Design review of the part shown in the three views and the two pictorial views. Dimensions are in mm from the part's minimum x, y and z. A direction names the side the tool comes from. Round coordinates to 2 decimals unless told otherwise and drop trailing zeros. Loops run counter-clockwise (first coordinate to the right, second up) from the corner with the lowest first, then second, coordinate; pieces in that order, holes last.
1) Take a section at D-D (z = 26). State the section outline as (x, y) points, then the cut area to 3 significant figures.
2) Wall thickness on L1, parallel to Y at x = 13.65, z = 3.5; L2, parallel to X at y = 25.75, z = 4; L3, parallel to Z at x = 8.75, y = 11.25: over which ranges is each line inside the solid? List them lowest first.
3) Take a section at A-A (z = 30.5). State the section outline as (x, y) points.
4) Take a section at C-C (y = 9.25). State the section outline as (x, z) points.
5) Tool access review of the marked faces 1, 2 and 3: name each direction out of +Z, -Z, +X, -X, +Y, -Y from which nothing blocks a thin tool from reaching the whole face with its end or side.
6) Take a section at B-B (y = 15). State the section outline as (x, z) points.
7) Mouldability with a two-part tool opening along X and no side actions: class the marked faces 4, 5 and 6 as pulls with the +X half, pulls with the -X half, needs draft (parallel to the pull), parting line crosses it, or undercut.
8) Insertion check: pin 1 (3.5 mm diameter, centred on x = 8, y = 17, fed in from +Z); pin 2 (6 mm diameter, centred on x = 5, z = 16, fed in from +Y); pin 3 (6 mm diameter, centred on x = 4.5, z = 16.5, fed in from -Y). Each pin has a flat end and moves straight along its axis. Give the tip position at first contact, or say it passes through.
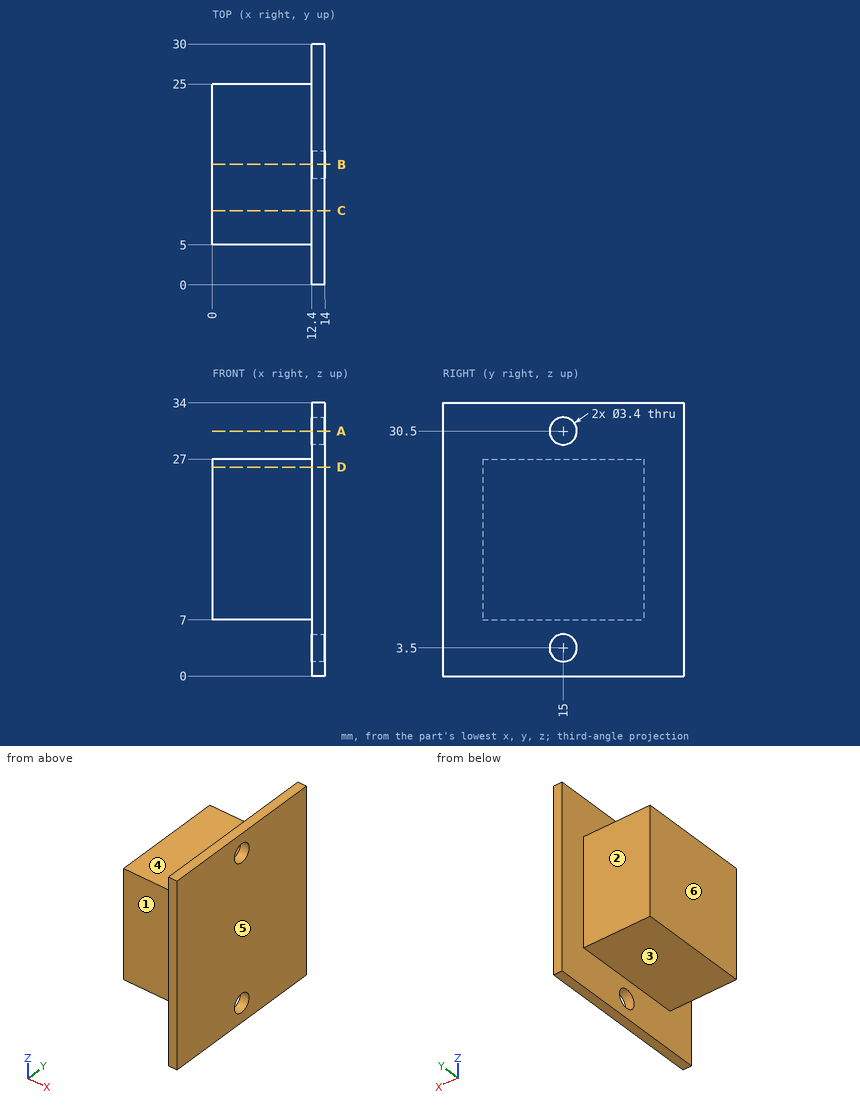
Response:
1. outline: (0, 5) - (12.4, 5) - (12.4, 0) - (14, 0) - (14, 30) - (12.4, 30) - (12.4, 25) - (0, 25) - close
1. area: 296 mm2
2. L1: y = 0 to 13.3, 16.7 to 30
2. L2: x = 12.4 to 14
2. L3: z = 7 to 27
3. outline: (12.4, 0) - (14, 0) - (14, 13.3) - (12.4, 13.3) - close; (12.4, 16.7) - (14, 16.7) - (14, 30) - (12.4, 30) - close
4. outline: (0, 7) - (12.4, 7) - (12.4, 0) - (14, 0) - (14, 34) - (12.4, 34) - (12.4, 27) - (0, 27) - close
5. face 1: +Z, -Z, -X, -Y
5. face 2: +Z, -Z, -X, +Y
5. face 3: -Z, -X, +Y, -Y
6. outline: (0, 7) - (12.4, 7) - (12.4, 5.2) - (14, 5.2) - (14, 28.8) - (12.4, 28.8) - (12.4, 27) - (0, 27) - close; (12.4, 0) - (14, 0) - (14, 1.8) - (12.4, 1.8) - close; (12.4, 32.2) - (14, 32.2) - (14, 34) - (12.4, 34) - close
7. face 4: needs draft
7. face 5: pulls with the +X half
7. face 6: pulls with the -X half
8. pin 1: stops at z = 27
8. pin 2: stops at y = 25
8. pin 3: stops at y = 5
